Source: three-view drawing plus pictorial views. Frame: mm from the lowest corner of the part. A direction names the side the tool comes from. Round coordinates to 2 decimals unless told otherwise and drop trailing zeros. Loops run counter-clockwise (first coordinate to the right, second up) from the corner with the lowest first, then second, coordinate; pieces in that order, holes last. Notation, with made-up numbers: M 59,-14.5 L 98,-14.5 A19 cw 98,-2.5 Z; hole C 63,9.5 d11. An arc over 180 degrees is marked long. Write each question's results on one line, items separated by ' | '.
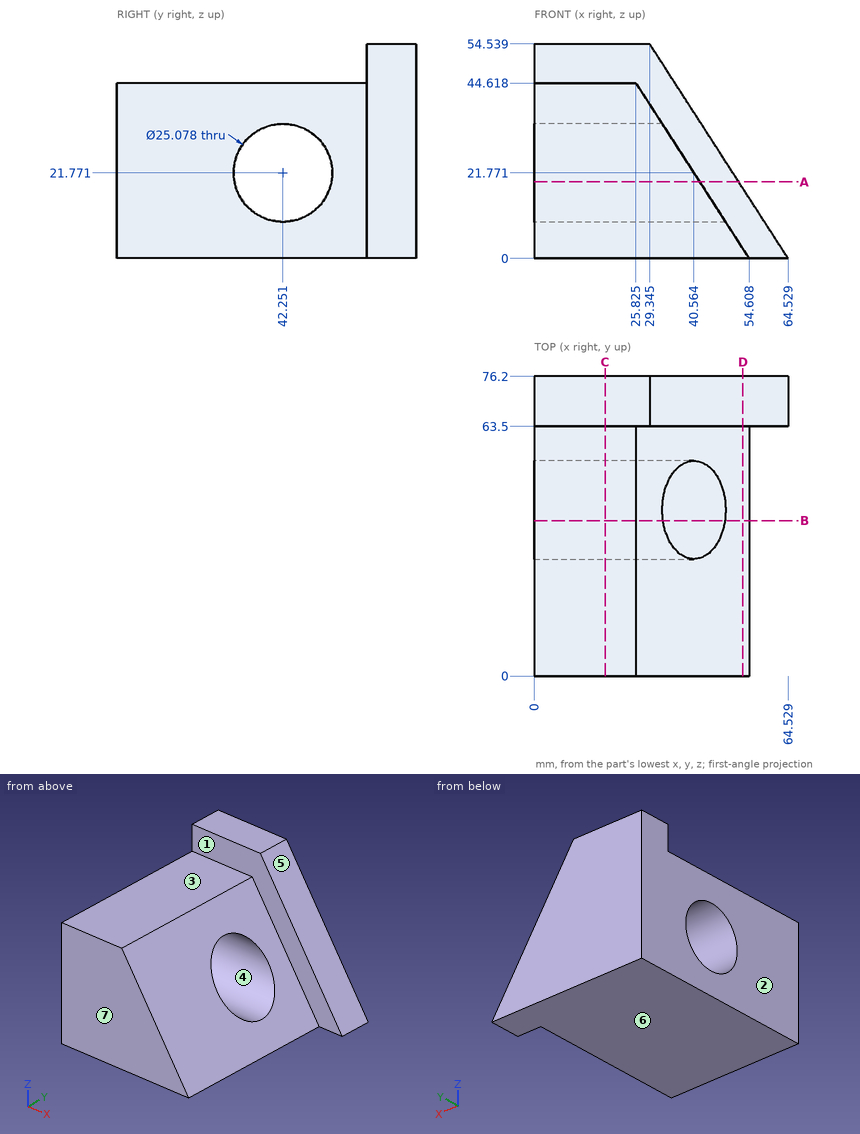
1. Section D-D (x = 53). Output: boundary loops of the cut face in (y, z), then the cut area to 3 significant figures.
Answer key:
outline: M 0,0 L 76.2,0 L 76.2,17.87 L 63.5,17.87 L 63.5,2.49 L 0,2.49 Z | area: 385 mm²
2. Section A-A (z = 19.5). Output: boundary loops of the cut face in (x, y), then the cut area to 3 significant figures.
Answer key:
outline: M 0,0 L 42.03,0 L 42.03,29.92 L 0,29.92 Z; M 0,54.58 L 42.03,54.58 L 42.03,63.5 L 51.95,63.5 L 51.95,76.2 L 0,76.2 Z | area: 2,290 mm²
3. Section B-B (y = 39.5). Output: boundary loops of the cut face in (x, z) (1 decimal), then the cut area to 3 significant figures.
Answer key:
outline: M 0,0 L 54.6,0 L 48.5,9.5 L 0,9.5 Z; M 0,34 L 32.7,34 L 25.8,44.6 L 0,44.6 Z | area: 802 mm²
4. Access query for the marked faces 1, 2 and 3. Directions: +Z, -Z, +X, -X, +Y, -Y. A direction counts if a zero-diameter tool reaches every point of the face in a straight line with its end or side. Return the directions, or none.
Answer key:
face 1: +Z, +X, -Y | face 2: +Z, -Z, -X, +Y, -Y | face 3: +Z, +X, -X, -Y
5. Section C-C (x = 18). Output: boundary loops of the cut face in (y, z), then the cut area to 3 significant figures.
Answer key:
outline: M 0,0 L 76.2,0 L 76.2,54.54 L 63.5,54.54 L 63.5,44.62 L 0,44.62 Z; hole C 42.25,21.77 d25.08 | area: 3,030 mm²
6. Ray query, probe 1 along Y at (x, z) = (30, 22) (1 decimal); probe 2 along Y at (x, z) = (42.5, 23.5); probe 3 along Y at (x, z) = (4, 12.5) (1 decimal). Return the intervals inside material, ascending.
Answer key:
probe 1: y = 0 to 29.7, 54.8 to 76.2 | probe 2: y = 63.5 to 76.2 | probe 3: y = 0 to 33.8, 50.7 to 76.2
7. Draft query along Z for the marked faces 4, 5, 6 and 7. Return one class per face: pulls with the +Z half, pulls with the -Z half, needs draft (parallel to the pull), parting line crosses it, or undercut.
Answer key:
face 4: undercut | face 5: pulls with the +Z half | face 6: pulls with the -Z half | face 7: needs draft
8. Pin query (flat end, axial travel): P1, Ø12, axis at x = 46.5, z = 48.5, coming from the -Y side; P2, Ø12, axis at y = 10, z = 35.5, coming from the +X side; P3, Ø10, axis at x = 26, y = 51, coming from the +Z side. Return the tip coordinate at first contact, or that it passes through.
Answer key:
P1: passes through | P2: stops at x = 35.58 | P3: stops at z = 44.62
